Here's how the part is built. I have some questions about the finished solid (model axes, mm). Face numbers are marked on the shaded views. A direction names the side the tool comes from. Coordinates: 2 decimals unless noted, no trailing zeros. Loops run counter-clockwise (first coordinate to the right, second up) from the corner with the lowest first, then second, coordinate; pieces in that order, holes last. Notation, with made-up numbers: M 62.25,42 L 87.25,42 A29 cw 87.25,63 Z; hole C 23,63 d4. An arc over 180 degrees is marked long. Use CSV: the item, a comma, the result in double quotes. Start each with the question number.
Q1. If we section it at B-B (x = 27): Please give me the cut outline in (y, z), and give its area (3 significant figures).
Q2. For pin 1 Ø1.7 at (y, z) = (-16, 9) entering from +X; pin 2 Ø1.8 at (x, z) = (54, 8.5) entering from -Y; pin 3 Ø10 at (x, y) = (32.5, -16) entering from +Z; pin 4 Ø3 at (x, y) = (41.28, -8) entering from -Z, each with a flat end and sliding along its axis, tell me the tip position at first contact or that it passes through.
Q3. If we section it at D-D (y = -27): Please give me the cut outline in (x, z).
Q4. If we mould it in two halves opening along Z, with no side actions, what happens to the marked faces 1, 2 and 3? For each: +Z half, -Z half, draft (parallel to the pull), parting line (faces both ways), or undercut.
Q5. Please list where these lines run through material, in increasing order: probe 1 along X at (y, z) = (-20.5, 14.75); probe 2 along X at (y, z) = (-21.5, 10.5); probe 3 along Y at (x, z) = (55, 9). Write a range as [from, to].
Q6. Which directions (+Z, -Z, +X, -X, +Y, -Y) give clear straight access to the entire face, cutting with the end or side of a thin tool? Please do the marked faces 4 and 5.
Q7. If we section it at C-C (z = 9): Please give me the cut outline in (x, y).
Q8. If we section it at A-A (y = -8): Please give me the cut outline in (x, z).
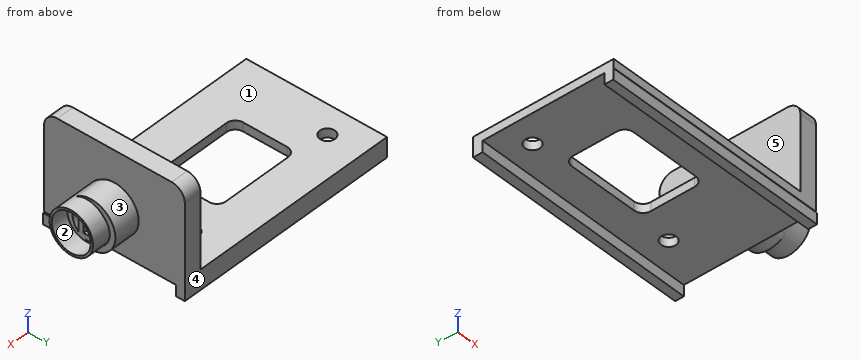
from build123d import *

# Parameters (mm, degrees)
SKETCH1_W           = 52
SKETCH1_H           = 32
BOSS_EXTRUDE1_DEPTH = 2
SKETCH2_W           = 4
SKETCH2_H           = 32
BOSS_EXTRUDE2_DEPTH = 20
FILLET1_R           = 3
SKETCH4_R           = 1.725
CUT_EXTRUDE2_DEPTH  = 2
SKETCH5_W           = 52.395546188
SKETCH5_H           = 2
BOSS_EXTRUDE3_DEPTH = 2.5
SKETCH6_W           = 20
SKETCH6_H           = 14
CUT_EXTRUDE3_DEPTH  = 2
SKETCH7_W           = 8.2
SKETCH7_H           = 5.8
SKETCH7_W_2         = 5.8
SKETCH7_H_2         = 3.4
BOSS_EXTRUDE4_DEPTH = 6
SKETCH10_R          = 4.93317494
SKETCH10_R_2        = 4.432714725
BOSS_EXTRUDE6_DEPTH = 10
SKETCH8_R           = 5.516570522
SKETCH8_R_2         = 4.25
BOSS_EXTRUDE5_DEPTH = 6
FILLET2_R           = 2


with BuildPart() as part:
    # Sketch1 → Boss-Extrude1 (new body)
    with BuildSketch(Plane.XY):
        with Locations((26, -16)):
            Rectangle(SKETCH1_W, SKETCH1_H)
    extrude(amount=BOSS_EXTRUDE1_DEPTH)

    # Sketch2 → Boss-Extrude2 (add)
    with BuildSketch(Plane(origin=(0, 0, 2), x_dir=(-1, 0, 0), z_dir=(0, 0, -1))):
        with Locations((-50, -16)):
            Rectangle(SKETCH2_W, SKETCH2_H)
    extrude(amount=-BOSS_EXTRUDE2_DEPTH)

    # Fillet1
    fillet1_edges = [part.edges().sort_by_distance(p)[0] for p in [
        (50, -32, 22),
        (50, 0, 22),
    ]]
    fillet(fillet1_edges, radius=FILLET1_R)

    # Sketch4 → Cut-Extrude2 (cut)
    with BuildSketch(Plane.XY.offset(2)):
        with Locations((41.277695867, -8)):
            Circle(SKETCH4_R)
        with Locations((6.277695867, -8)):
            Circle(SKETCH4_R)
    extrude(amount=-CUT_EXTRUDE2_DEPTH, mode=Mode.SUBTRACT)

    # Sketch5 → Boss-Extrude3 (add)
    with BuildSketch(Plane(origin=(0, 0, 0), x_dir=(-1, 0, 0), z_dir=(0, 0, -1))):
        with Locations((-26.197773094, -30.904147889)):
            Rectangle(SKETCH5_W, SKETCH5_H)
        Polygon((-52, -1.965960074), (0, -2.193486325), (0, 0), (-52, 0), align=None)
    extrude(amount=BOSS_EXTRUDE3_DEPTH)

    # Sketch6 → Cut-Extrude3 (cut)
    with BuildSketch(Plane.XY.offset(2)):
        with Locations((23.277695867, -16)):
            Rectangle(SKETCH6_W, SKETCH6_H)
    extrude(amount=-CUT_EXTRUDE3_DEPTH, mode=Mode.SUBTRACT)

    # Sketch7 → Boss-Extrude4 (add)
    with BuildSketch(Plane(origin=(52, 0, 0), x_dir=(0, 0, -1), z_dir=(1, 0, 0))):
        with Locations((-9.5, -16)):
            Rectangle(SKETCH7_W, SKETCH7_H)
        with Locations((-9.5, -16)):
            Rectangle(SKETCH7_W_2, SKETCH7_H_2, mode=Mode.SUBTRACT)
    extrude(amount=BOSS_EXTRUDE4_DEPTH)

    # Sketch10 → Boss-Extrude6 (add)
    with BuildSketch(Plane(origin=(52, 0, 0), x_dir=(0, 0, -1), z_dir=(1, 0, 0))):
        with Locations(Location((-9.443010808, -16.994711926, 0), (0, 0, 147.422084195))):
            Circle(SKETCH10_R)
        with Locations(Location((-9.443010808, -16.994711926, 0), (0, 0, 159.684920178))):
            Circle(SKETCH10_R_2, mode=Mode.SUBTRACT)
    extrude(amount=BOSS_EXTRUDE6_DEPTH)

    # Sketch8 → Boss-Extrude5 (add)
    with BuildSketch(Plane(origin=(52, 0, 0), x_dir=(0, 0, -1), z_dir=(1, 0, 0))):
        with Locations((-9.395508103, -16)):
            Circle(SKETCH8_R)
        with Locations((-9.395508103, -16)):
            Circle(SKETCH8_R_2, mode=Mode.SUBTRACT)
    extrude(amount=BOSS_EXTRUDE5_DEPTH)

    # Fillet2
    fillet2_edges = [part.edges().sort_by_distance(p)[0] for p in [
        (33.277695867, -9, 1),
        (33.277695867, -23, 1),
        (13.277695867, -23, 1),
        (13.277695867, -9, 1),
    ]]
    fillet(fillet2_edges, radius=FILLET2_R)


solid = part.part
Results below:
1,outline,"M -32,0 L -31.9,0 L -31.9,-2.5 L -29.9,-2.5 L -29.9,0 L -23,0 L -23,2 L -32,2 Z; M -9,0 L -2.08,0 L -2.08,-2.5 L 0,-2.5 L 0,2 L -9,2 Z"
1,area,"46.2 mm^2"
2,pin 1,"x = 52"
2,pin 2,"y = -21.93"
2,pin 3,"z = 2"
2,pin 4,"through"
3,outline,"M 0,0 L 52,0 L 52,22 L 48,22 L 48,2 L 0,2 Z"
4,face 1,"+Z half"
4,face 2,"undercut"
4,face 3,"parting line"
5,probe 1,"[48, 52]"
5,probe 2,"[48, 62]"
5,probe 3,"[-21.91, -20.23], [-18.9, -17.7], [-14.3, -13.1], [-12.58, -12.08], [-11.77, -10.5]"
6,face 4,"+Z, -Z, +X, -X, +Y"
6,face 5,"+Z, -X, +Y, -Y"
7,outline,"M 48,-32 L 52,-32 L 52,-21.91 L 62,-21.91 L 62,-21.41 L 58,-21.41 L 58,-20.23 L 52,-20.23 L 52,-18.9 L 58,-18.9 L 58,-17.7 L 52,-17.7 L 52,-14.3 L 58,-14.3 L 58,-13.1 L 52,-13.1 L 52,-12.58 L 62,-12.58 L 62,-12.08 L 52,-12.08 L 52,-11.77 L 58,-11.77 L 58,-10.5 L 52,-10.5 L 52,0 L 48,0 Z"
8,outline,"M 0,0 L 4.55,0 L 4.55,2 L 0,2 Z; M 8,0 L 39.55,0 L 39.55,2 L 8,2 Z; M 43,0 L 52,0 L 52,22 L 48,22 L 48,2 L 43,2 Z"
